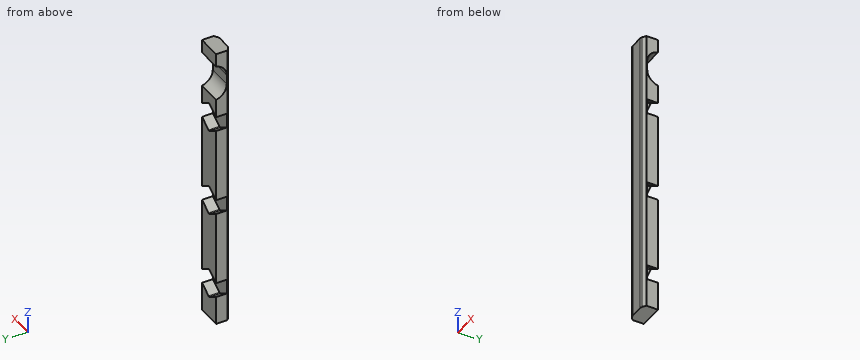
from build123d import *

# Parameters (mm, degrees)
BOSS_EXTRUDE1_DEPTH = 65
FILLET3_R           = 1
FILLET4_R           = 1
CUT_EXTRUDE1_DEPTH  = 2.4
LPATTERN1_COUNT     = 3
LPATTERN1_PITCH     = 20
SKETCH3_W           = 5.4
SKETCH3_H           = 8
CUT_EXTRUDE2_DEPTH  = 2.4
FILLET5_R           = 3
FILLET6_R           = 0.35


with BuildPart() as part:
    # Sketch1 → Boss-Extrude1 (new body)
    with BuildSketch(Plane.XY):
        Polygon((0, 0), (3.4, 0), (4.4, 0.663324958), (4.4, 3.263324958), (-1, 3.263324958), (-1, 0.663324958), align=None)
    extrude(amount=BOSS_EXTRUDE1_DEPTH)

    # Fillet3
    fillet3_edges = [part.edges().sort_by_distance(p)[0] for p in [
        (3.4, 0, 32.5),
    ]]
    fillet(fillet3_edges, radius=FILLET3_R)

    # Fillet4
    fillet4_edges = [part.edges().sort_by_distance(p)[0] for p in [
        (0, 0, 32.5),
    ]]
    fillet(fillet4_edges, radius=FILLET4_R)

    # Sketch2 → Cut-Extrude1 (cut)
    with BuildSketch(Plane(origin=(0, 3.263324958, 0), x_dir=(1, 0, 0), z_dir=(0, 1, 0))):
        Polygon((4.4, -9.81), (4.4, -6.48), (1.7, -4.8), (-1, -6.48), (-1, -9.81), (1.7, -11.49), align=None)
    cut_extrude1 = extrude(amount=-CUT_EXTRUDE1_DEPTH, mode=Mode.SUBTRACT)

    # LPattern1: Cut-Extrude1 ×3
    with Locations(*[(0, 0, i * LPATTERN1_PITCH) for i in range(1, LPATTERN1_COUNT)]):
        add(cut_extrude1, mode=Mode.SUBTRACT)

    # Sketch3 → Cut-Extrude2 (cut)
    with BuildSketch(Plane(origin=(0, 3.263324958, 0), x_dir=(1, 0, 0), z_dir=(0, 1, 0))):
        with Locations((1.7, -58)):
            Rectangle(SKETCH3_W, SKETCH3_H)
    extrude(amount=-CUT_EXTRUDE2_DEPTH, mode=Mode.SUBTRACT)

    # Fillet5
    # the kernel refuses this fillet: 3 mm, written as the material it adds along each edge
    with BuildSketch(Plane(origin=(4.4, 0.863324958, 54), x_dir=(0, 0, 1), z_dir=(-1, 0, 0))) as fillet5_piece_1:
        with BuildLine():
            CenterArc((2.939387691, 3), FILLET5_R, 191.536959033, 78.463040967)
            Line((0, 2.4), (-0.058787754, 2.388))
            ThreePointArc((-0.058787754, 2.388), (-0.06, 1.2), (-0.06, 0))
            Line((-0.06, 0), (0, -0.06))
            Line((0, -0.06), (2.939387691, -0.06))
            Line((2.939387691, -0.06), (2.939387691, 0))
        make_face()
    extrude(amount=5.4)
    with BuildSketch(Plane(origin=(-1, 0.863324958, 62), x_dir=(0, 1.0, -1.5483910450100627e-12), z_dir=(1, 0, 0))) as fillet5_piece_2:
        with BuildLine():
            CenterArc((3, -2.939387691), FILLET5_R, 101.536959033, 78.463040967)
            Line((0, -2.939387691), (-0.06, -2.939387691))
            Line((-0.06, -2.939387691), (-0.06, 0))
            Line((-0.06, 0), (0, 0.06))
            ThreePointArc((0, 0.06), (1.2, 0.06), (2.388, 0.058787754))
            Line((2.388, 0.058787754), (2.4, 0))
        make_face()
    extrude(amount=5.4)

    # Fillet6
    fillet6_edges = [part.edges().sort_by_distance(p)[0] for p in [
        (1.7, 2.063324958, 11.49),
        (1.7, 2.063324958, 4.8),
        (1.7, 2.063324958, 31.49),
        (1.7, 2.063324958, 24.8),
        (1.7, 2.063324958, 51.49),
        (1.7, 2.063324958, 44.8),
    ]]
    fillet(fillet6_edges, radius=FILLET6_R)


solid = part.part
Could you check a few things on this model? Use its own coordinates, in mm. Coordinates: 2 decimals unless noted, no trailing zeros. Order: outer loops, then holes, each group sorted by start corner. A loop starts at its lowest first (then second) coordinate and runs counter-clockwise, first axis right, second up. Notation, with made-up numbers: (13.25, 17.25) - (18.25, 17.25) arc R11 cw to (18.25, 36.25) - close; hole circle Ø6 at (46, -21). An arc over 180 degrees is marked (long way). Answer in a Markdown table with one row per item. Add a question column.
(1) If we section it at C-C, the plane z = 45.5: Please give me the cut outline in (x, y) (3 decimals).
(2) I need wall thicknesses on L1, parallel to Z at x = 3.95, y = 1.65; L2, parallel to Z at x = 1.65, y = 1.35; L3, parallel to Y at x = -0.25, z = 38.5. Which ranges of each line are inside material? Lowest first, please.
(3) If we section it at B-B, the plane y = 2.25: State how many separate pieces and enclosed holes the cut face has, then the cut area to 3 significant figures.
(4) If we section it at A-A, the plane z = 35: Please give me the cut outline in (x, y), then the cut area to 3 significant figures.
(5) Will this pin go through, and if not, where does the flat tip stop? pin 1 (1.1 mm diameter, centred on x = 2, z = 58, fed in from +Y).
Results are:
| question | item | result |
|---|---|---|
| 1 | outline | (-1, 0.663) - (-0.251, 0.167) arc R1 ccw to (0.302, 0) - (3.098, 0) arc R1 ccw to (3.651, 0.167) - (4.4, 0.663) - (4.4, 3.263) - (2.825, 3.263) - (2.825, 0.863) - (0.575, 0.863) - (0.575, 3.263) - (-1, 3.263) - close |
| 2 | L1 | z = 0 to 6.2, 10.09 to 26.2, 30.09 to 46.2, 50.09 to 54.91, 61.09 to 65 |
| 2 | L2 | z = 0 to 4.87, 11.42 to 24.87, 31.42 to 44.87, 51.42 to 55.3, 60.7 to 65 |
| 2 | L3 | y = 0.17 to 3.26 |
| 3 | separate pieces | 5 |
| 3 | enclosed holes | 0 |
| 3 | area | 231 mm2 |
| 4 | outline | (-1, 0.66) - (-0.25, 0.17) arc R1 ccw to (0.3, 0) - (3.1, 0) arc R1 ccw to (3.65, 0.17) - (4.4, 0.66) - (4.4, 3.26) - (-1, 3.26) - close |
| 4 | area | 16.9 mm2 |
| 5 | pin 1 | stops at y = 0.86 |
